Here's the drawing with two shaded views (mm, measured from the low corner). I have some questions. A direction names the side the tool comes from. Round coordinates to 2 decimals unless told otherwise and drop trailing zeros. Loops run counter-clockwise (first coordinate to the right, second up) from the corner with the lowest first, then second, coordinate; pieces in that order, holes last. Notation, with made-up numbers: (65, 54) - (104, 54) arc R32 ccw to (104, 90) - close; hole circle Ø10 at (-8.5, -36.5). An arc over 180 degrees is marked (long way). Use one line per item in the form item = value.
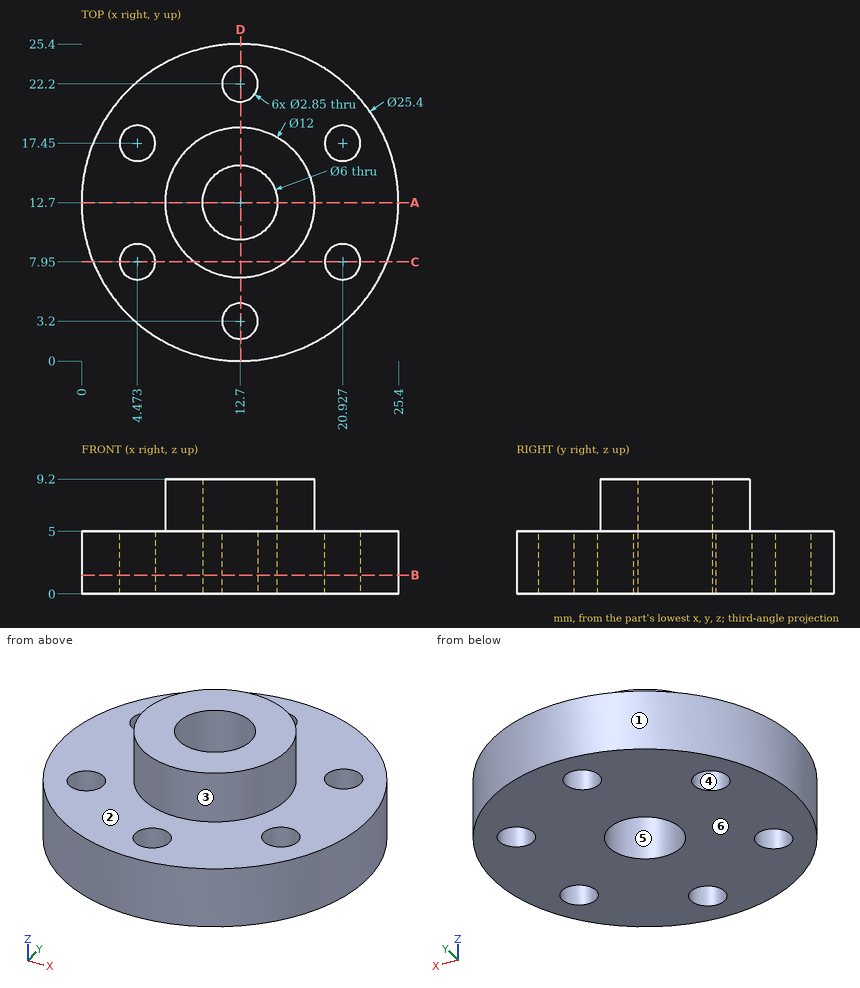
1. Please list where these lines run through material, in increasing order: line 1 along Y through (x, z) = (12.7, 2) (1 decimal); line 2 along Y through (x, z) = (4.5, 2.75) (1 decimal); line 3 along X through (y, z) = (8, 0.5).
Solution:
line_1 = 0 to 1.8, 4.6 to 9.7, 15.7 to 20.8, 23.6 to 25.4
line_2 = 3 to 6.5, 9.4 to 16, 18.9 to 22.4
line_3 = 0.9 to 3.05, 5.9 to 19.5, 22.35 to 24.5
2. If we section it at A-A, the plane y = 12.7: Write out the boundary of the cut face in (x, z), plus the area to 3 significant figures.
Solution:
outline = (0, 0) - (9.7, 0) - (9.7, 9.2) - (6.7, 9.2) - (6.7, 5) - (0, 5) - close; (15.7, 0) - (25.4, 0) - (25.4, 5) - (18.7, 5) - (18.7, 9.2) - (15.7, 9.2) - close
area = 122 mm^2
3. On a 3-axis mill with a long thin cutter (end or side, diameter ignored), from which of +Z, -Z, +X, -X, +Y, -Y can I reach the whole of each face in a straight line? I mean the marked faces 1 and 2. Say none if no direction works.
Solution:
face_1 = +Z, -Z
face_2 = +Z
4. For P1, Ø1.7, axis at x = 4.47, y = 17.45, coming from the +Z side; P2, Ø4.5, axis at x = 12.7, y = 3.2, coming from the +Z side; P3, Ø1, axis at x = 11, z = 2, coming from the +Y side; P4, Ø3, axis at y = 19, z = 4, coming from the +X side, each with a flat end and sliding along its axis, tell me the tip position at first contact or that it passes through.
Solution:
P1 = through
P2 = 5
P3 = 25.34
P4 = 24.46
5. If we section it at D-D, the plane x = 12.75: Write out the boundary of the cut face in (y, z).
Solution:
outline = (0, 0) - (1.78, 0) - (1.78, 5) - (0, 5) - close; (4.62, 0) - (9.7, 0) - (9.7, 9.2) - (6.7, 9.2) - (6.7, 5) - (4.62, 5) - close; (15.7, 0) - (20.78, 0) - (20.78, 5) - (18.7, 5) - (18.7, 9.2) - (15.7, 9.2) - close; (23.62, 0) - (25.4, 0) - (25.4, 5) - (23.62, 5) - close
6. We'd pull the mould along Y, two halves only. Please class the marked faces 3, 4, 5 and 6: +Y half, -Y half, draft (parallel to the pull), parting line (faces both ways), or undercut.
Solution:
face_3 = parting line
face_4 = undercut
face_5 = undercut
face_6 = draft
7. If we section it at B-B, the plane z = 1.5: Count the separate pieces of the cut face and the enclosed holes in it, plus the area to 3 significant figures.
Solution:
separate_pieces = 1
enclosed_holes = 7
area = 440 mm^2
8. If we section it at C-C, the plane y = 7.95: Write out the boundary of the cut face in (x, z), plus the area to 3 significant figures.
Solution:
outline = (0.92, 0) - (3.05, 0) - (3.05, 5) - (0.92, 5) - close; (5.9, 0) - (19.5, 0) - (19.5, 5) - (16.37, 5) - (16.37, 9.2) - (9.03, 9.2) - (9.03, 5) - (5.9, 5) - close; (22.35, 0) - (24.48, 0) - (24.48, 5) - (22.35, 5) - close
area = 120 mm^2
